Verification items for this drawing (mm, ordinates from the low corner). Round coordinates to 2 decimals unless told otherwise and drop trailing zeros. Loops run counter-clockwise (first coordinate to the right, second up) from the corner with the lowest first, then second, coordinate; pieces in that order, holes last. Notation, with made-up numbers: M 5,43 L 55,43 A15 cw 55,54 Z; hole C 32,-20.75 d9. An arc over 180 degrees is marked long. Write item = value, one per line. Start each with the question number.
(1) Cross-section at D-D on x = 196. Record the boundary of the cut face in (y, z), plus the area to 3 significant figures.
(2) Cross-section at C-C on y = 51.5. Record the boundary of the cut face in (x, z).
(3) Cross-section at A-A on x = 31.5. Record the boundary of the cut face in (y, z), plus the area to 3 significant figures.
(4) Scan lines: L1, parallel to Y at x = 115.57, z = 3.1; L2, parallel to X at y = 81.28, z = 2.4; L3, parallel to Y at x = 2.54, z = 2.8. Record each from-to range of solid material in increasing order. Write a range as from..to.
(5) Cross-section at B-B on z = 1. Record the boundary of the cut face in (x, y), plus the area to 3 significant figures.
(6) Go/stop test with flat-tipped pins: P1, Ø1.5, axis at y = 106.5, z = 3.5, coming from the -X side; P2, Ø2.5, axis at x = 29, z = 2.5, coming from the -Y side; P3, Ø2.5, axis at y = 24.5, z = 3.5, coming from the +X side; P4, Ø2.5, axis at y = 160.5, z = 3.5, coming from the +X side. Record where each tip stops, or that it passes through.
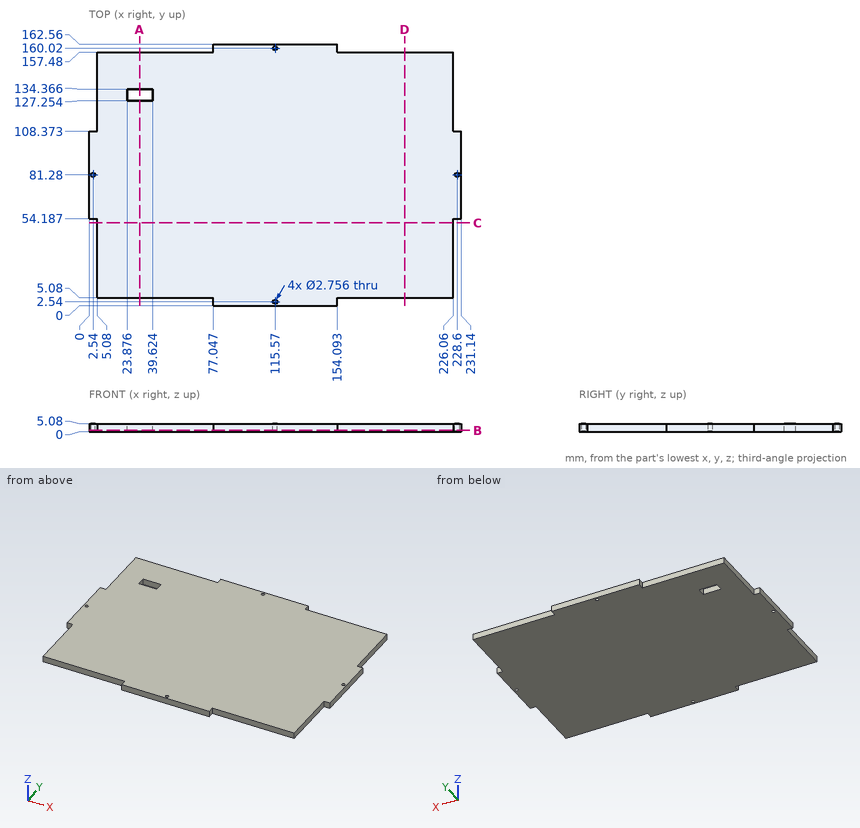
Result:
q1.outline = M 5.08,0 L 157.48,0 L 157.48,5.08 L 5.08,5.08 Z
q1.area = 774 mm^2
q2.outline = M 5.08,0 L 226.06,0 L 226.06,5.08 L 5.08,5.08 Z
q3.outline = M 5.08,0 L 127.25,0 L 127.25,5.08 L 5.08,5.08 Z; M 134.37,0 L 157.48,0 L 157.48,5.08 L 134.37,5.08 Z
q3.area = 738 mm^2
q4.L1 = 0..1.16, 3.92..158.64, 161.4..162.56
q4.L2 = 0..1.16, 3.92..227.22, 229.98..231.14
q4.L3 = 54.19..79.9, 82.66..108.37
q5.outline = M 0,54.19 L 5.08,54.19 L 5.08,5.08 L 77.05,5.08 L 77.05,0 L 154.09,0 L 154.09,5.08 L 226.06,5.08 L 226.06,54.19 L 231.14,54.19 L 231.14,108.37 L 226.06,108.37 L 226.06,157.48 L 154.09,157.48 L 154.09,162.56 L 77.05,162.56 L 77.05,157.48 L 5.08,157.48 L 5.08,108.37 L 0,108.37 Z; hole C 2.54,81.28 d2.76; hole M 23.88,127.25 L 39.62,127.25 L 39.62,134.37 L 23.88,134.37 Z; hole C 115.57,2.54 d2.76; hole C 115.57,160.02 d2.76; hole C 228.6,81.28 d2.76
q5.area = 34,900 mm^2
q6.P1 = 0
q6.P2 = 5.08
q6.P3 = 226.06
q6.P4 = 154.09
